The drawing under review shows one solid part. Ordinate dimensions are in mm from its lowest x, y, z. A direction names the side the tool comes from. Give positions to 0.01 mm unless a question says otherwise; leave off trailing zeros. Write each loop counter-clockwise with the first axis right and the second up, starting at its lowest first coordinate (ties: lowest second). Pieces come first, ordered by that corner, then holes. Notation, with made-up numbers: M 61,66 L 114,66 A23 ccw 114,100 Z; hole C 71.25,81 d8. An arc over 180 degrees is marked long. Write item = value, one per line. Start each with the question number.
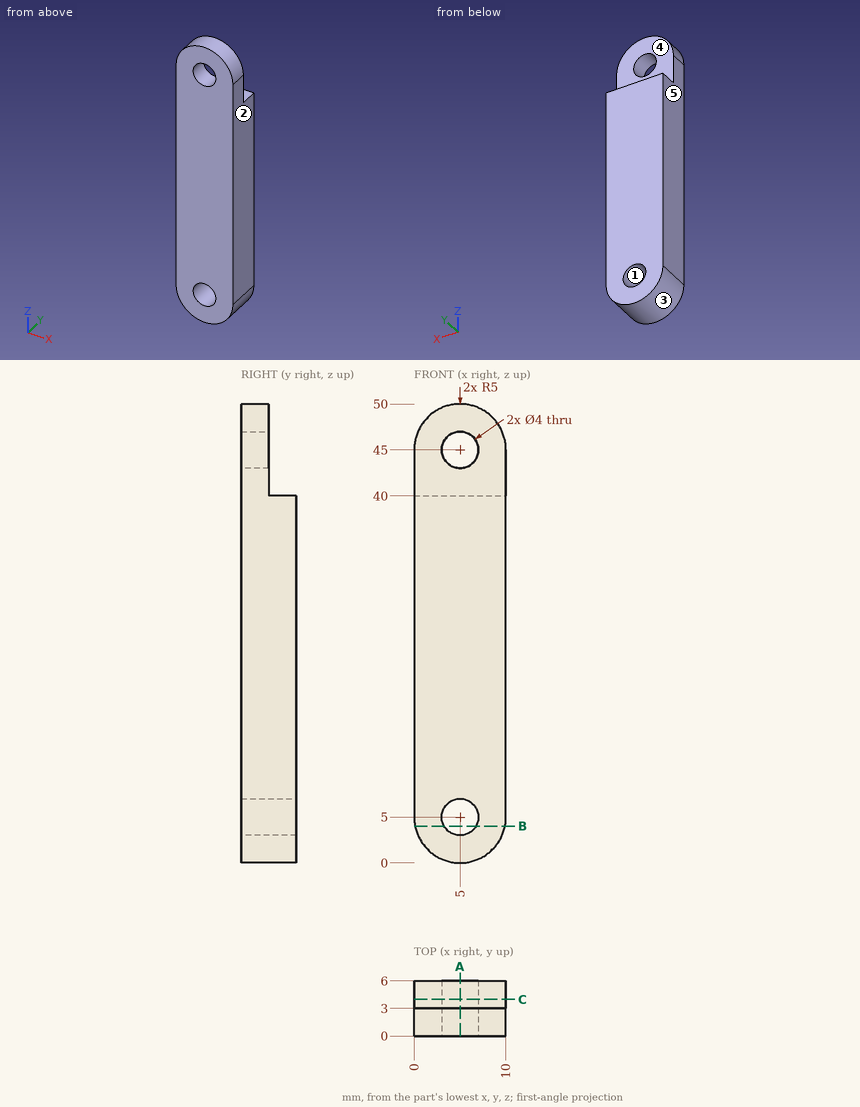
Item 1: The part is to be moulded in two halves that separate along Z. For the marked faces 1, 2 and 3, say which applies: released by +Z, released by -Z, zero draft, split by the parting line, or undercut.
Item 2: We need section A-A, the plane x = 5. Write out the cut boundary in (y, z), and give its area (3 significant figures).
Item 3: We need section C-C, the plane y = 4. Write out the cut boundary in (x, z).
Item 4: Clearance check with flat-ended pins moving along their axes: P1, Ø3.5, axis at x = 6, y = 4.5, coming from the +Z side; P2, Ø3, axis at x = 5, z = 45, coming from the -Y side; P3, Ø3, axis at x = 6.5, z = 47.5, coming from the +Y side. State where each tip first meets the part, or that it passes through.
Item 5: For the marked faces 4 and 5, list the 3-axis set-ups (+Z, -Z, +X, -X, +Y, -Y) from which the entire face can be reached by the end or side of a thin tool; tool diameter is ignored.
Item 6: To check wall thickness, follow probe 1 along Z at (x, y) = (4, 1.2); probe 2 along X at (y, z) = (4.35, 5); probe 3 along Y at (x, z) = (6.25, 42). State the ranges of each line that lie inside material, in increasing order. Write a range as [from, to].
Item 7: We need section B-B, the plane z = 4. Write out the cut boundary in (x, y).
Worked out:
q1.face_1 = undercut
q1.face_2 = zero draft
q1.face_3 = released by -Z
q2.outline = M 0,0 L 6,0 L 6,3 L 0,3 Z; M 0,7 L 6,7 L 6,40 L 3,40 L 3,43 L 0,43 Z; M 0,47 L 3,47 L 3,50 L 0,50 Z
q2.area = 234 mm²
q3.outline = M 0,5 A5 ccw 10,5 L 10,40 L 0,40 Z; hole C 5,5 d4
q4.P1 = 50
q4.P2 = through
q4.P3 = 3
q5.face_4 = +Z, +X, -X, +Y
q5.face_5 = +Z, -Z, -X, +Y, -Y
q6.probe_1 = [0.1, 3.27], [6.73, 43.27], [46.73, 49.9]
q6.probe_2 = [0, 3], [7, 10]
q6.probe_3 = [0, 3]
q7.outline = M 0.1,0 L 3.27,0 L 3.27,6 L 0.1,6 Z; M 6.73,0 L 9.9,0 L 9.9,6 L 6.73,6 Z
